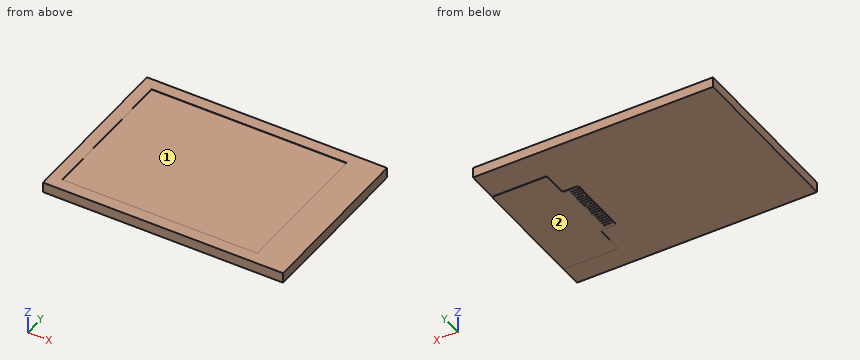
```python
from build123d import *

# Parameters (mm, degrees)
SKETCH_W            = 60.26
SKETCH_H            = 42.72
PAD_DEPTH           = 2.6
SKETCH001_W         = 48.96
SKETCH001_H         = 36.72
POCKET_DEPTH        = 0.1
PAD001_DEPTH        = 0.1
FILLET_R            = 0.5
SKETCH003_W         = 2.5
SKETCH003_H         = 0.4
PAD002_DEPTH        = 0.05
LINEARPATTERN_COUNT = 18
LINEARPATTERN_PITCH = 0.8


with BuildPart() as part:
    # Sketch → Pad (new body)
    with BuildSketch(Plane.XY):
        with Locations((30.13, 21.36)):
            Rectangle(SKETCH_W, SKETCH_H)
    extrude(amount=PAD_DEPTH)

    # Sketch001 (on Face6 of Pad) → Pocket (cut)
    with BuildSketch(Plane.XY.offset(2.6)):
        with Locations((27.48, 21.36)):
            Rectangle(SKETCH001_W, SKETCH001_H)
    extrude(amount=-POCKET_DEPTH, mode=Mode.SUBTRACT)

    # Sketch002 (on Face4 of Pocket) → Pad001 (join)
    with BuildSketch(Plane(origin=(0, 0, 0), x_dir=(1, 0, 0), z_dir=(0, 0, -1))):
        Polygon((60.26, -5.6), (46.5, -5.6), (46.5, -12.9), (42.5, -12.9), (42.5, -28.5), (46.5, -28.5), (46.5, -34.9), (60.26, -34.9), align=None)
    extrude(amount=PAD001_DEPTH)

    # Fillet
    fillet_edges = [part.edges().sort_by_distance(p)[0] for p in [
        (46.5, 5.6, -0.05),
        (46.5, 12.9, -0.05),
        (42.5, 12.9, -0.05),
        (42.5, 28.5, -0.05),
        (46.5, 28.5, -0.05),
        (46.5, 34.9, -0.05),
        (60.26, 34.9, -0.05),
        (60.26, 5.6, -0.05),
    ]]
    fillet(fillet_edges, radius=FILLET_R)

    # Sketch003 (on Face22 of Fillet) → Pad002 (join)
    with BuildSketch(Plane(origin=(0, 0, -0.1), x_dir=(1, 0, 0), z_dir=(0, 0, -1))):
        with Locations((43.75, -13.9)):
            Rectangle(SKETCH003_W, SKETCH003_H)
    pad002 = extrude(amount=PAD002_DEPTH)

    # LinearPattern: Pad002 ×18
    with Locations(*[(0, i * LINEARPATTERN_PITCH, 0) for i in range(1, LINEARPATTERN_COUNT)]):
        add(pad002)


solid = part.part
```
The model under review builds one solid part; all positions refer to its coordinate system, in mm. Face numbers are marked on the shaded views. Give positions to 0.01 mm unless a question says otherwise; leave off trailing zeros. Write each loop counter-clockwise with the first axis right and the second up, starting at its lowest first coordinate (ties: lowest second). Pieces come first, ordered by that corner, then holes. Notation, with made-up numbers: M 1,83 L 60,83 A26 ccw 60,113 Z; hole C 53,-14.5 d3. An arc over 180 degrees is marked long. Write each question's results on one line, items separated by ' | '. Start each with the question number.
1. For probe 1 along Z at (x, y) = (54, 21); probe 2 along Z at (x, y) = (48, 3.5), list the stretches that pass through material, from the lowest coordinate up. Write a range as [from, to].
2. Mouldability with a two-part tool opening along X and no side actions: class the marked faces 1 and 2 as released by +X, released by -X, zero draft, split by the parting line, or undercut.
3. We need section B-B (y = 39). Write out the cut boundary in (x, z), and give its area (3 significant figures).
4. We need section A-A (x = 33). Write out the cut boundary in (y, z).
5. We need section C-C (y = 30). Write out the cut boundary in (x, z).
6. Insertion check: pin 1 Ø1.5 at (x, y) = (42.5, 35) entering from +Z; pin 2 Ø6 at (x, y) = (23.5, 21) entering from -Z. Each pin has a flat end and moves straight along its axis. Give the tip position at first contact, or say it passes through.
Results found:
1) probe 1: z = [-0.1, 2.6] | probe 2: z = [0, 2.5]
2) face 1: undercut | face 2: zero draft
3) outline: M 0,0 L 60.26,0 L 60.26,2.6 L 51.96,2.6 L 51.96,2.5 L 3,2.5 L 3,2.6 L 0,2.6 Z | area: 152 mm^2
4) outline: M 0,0 L 42.72,0 L 42.72,2.6 L 39.72,2.6 L 39.72,2.5 L 3,2.5 L 3,2.6 L 0,2.6 Z
5) outline: M 0,0 L 46.5,0 L 46.5,-0.1 L 60.26,-0.1 L 60.26,2.6 L 51.96,2.6 L 51.96,2.5 L 3,2.5 L 3,2.6 L 0,2.6 Z
6) pin 1: stops at z = 2.5 | pin 2: stops at z = 0
